from build123d import *

# Parameters (mm, degrees)
SKETCH_1_W               = 40
SKETCH_1_H               = 40.8
SKETCH_1_R               = 8
SKETCH_1_R_2             = 2.025
EXTRUDE_1_DEPTH          = 6
CUT_EXTRUDE_1_DEPTH      = 32.511267826
CUT_EXTRUDE_1_DEPTH_BACK = 32.511267826
SKETCH_2_R               = 1.5


with BuildPart() as part:
    # 草图1 → 凸台-拉伸1 (new body)
    with BuildSketch(Plane(origin=(0, 0, 0), x_dir=(0, 0, -1), z_dir=(1, 0, 0))):
        with Locations((0, 3.2)):
            Rectangle(SKETCH_1_W, SKETCH_1_H)
        Circle(SKETCH_1_R, mode=Mode.SUBTRACT)
        with Locations((-8.838834765, 8.838834765)):
            Circle(SKETCH_1_R_2, mode=Mode.SUBTRACT)
        with Locations((8.838834765, 8.838834765)):
            Circle(SKETCH_1_R_2, mode=Mode.SUBTRACT)
        with Locations((8.838834765, -8.838834765)):
            Circle(SKETCH_1_R_2, mode=Mode.SUBTRACT)
        with Locations((-8.838834765, -8.838834765)):
            Circle(SKETCH_1_R_2, mode=Mode.SUBTRACT)
    extrude(amount=EXTRUDE_1_DEPTH)

    # 草图2 → 切除-拉伸1 (cut, two sides: drawn at the far end of the back side and taken through both)
    with BuildSketch(Plane(origin=(0, 0, 0), x_dir=(1, 0, 0), z_dir=(0, 1, 0)).offset(-CUT_EXTRUDE_1_DEPTH_BACK)):
        with Locations(Location((3, 15, 0), (0, 0, 270))):
            Circle(SKETCH_2_R)
        with Locations(Location((3, -15, 0), (0, 0, 270))):
            Circle(SKETCH_2_R)
    extrude(amount=CUT_EXTRUDE_1_DEPTH + CUT_EXTRUDE_1_DEPTH_BACK, mode=Mode.SUBTRACT)


solid = part.part
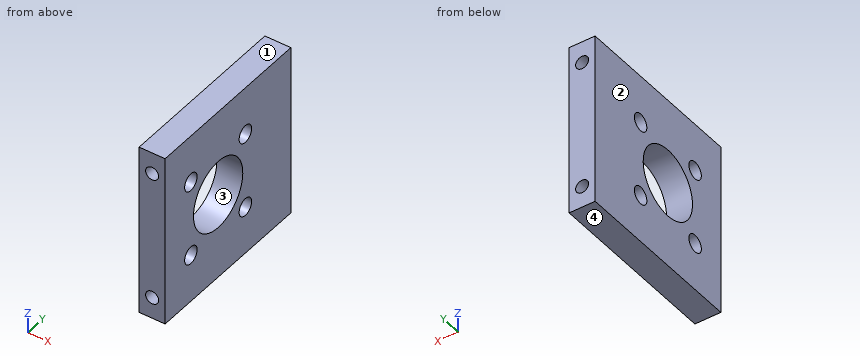
The model under review builds one solid part; all positions refer to its coordinate system, in mm. Face numbers are marked on the shaded views. Give positions to 0.01 mm unless a question says otherwise; leave off trailing zeros. Loops run counter-clockwise (first coordinate to the right, second up) from the corner with the lowest first, then second, coordinate; pieces in that order, holes last. Notation, with made-up numbers: (11.25, 28) -> (36.25, 28) arc R21 cw to (36.25, 40) -> close; hole circle Ø2 at (86, 22.25). An arc over 180 degrees is marked (long way). Answer as a JSON object with one key per item and string values. Group by question number.
Q1. Insertion check: pin 1 (2.5 mm diameter, centred on x = 3, z = 15, fed in from -Y). The pin has a flat end and moves straight along its axis. Give the tip position at first contact, or say it passes through.
Q2. Take a section at C-C (x = 3). Write out the cut boundary in (y, z) (3 decimals), plus the area to 3 significant figures.
Q3. Wall thickness on line 1 along Z through (x, y) = (3.1, 19); line 2 along Y through (x, z) = (2.5, 9); line 3 along Z through (x, y) = (5.45, -9): over which ranges is each line inside the solid? List them lowest first.
Q4. Draft analysis for pull direction Z (two halves, no side actions). For the marked faces 1, 2, 3 and 4, state which applies: pulls with the +Z half, pulls with the -Z half, needs draft (parallel to the pull), parting line crosses it, or undercut.
Q5. Take a section at D-D (x = 5.1). Write out the cut boundary in (y, z) (3 decimals), plus the area to 3 significant figures.
Q6. Take a section at A-A (y = 2.5). Write out the cut boundary in (x, z).
Q7. Take a section at B-B (z = 15). Write out the cut boundary in (x, y).
Answer below:
{
 "1": {"pin 1": "passes through"},
 "2": {"outline": "(-17.2, -20) -> (23.6, -20) -> (23.6, -16.5) -> (-17.2, -16.5) -> close; (-17.2, -13.5) -> (23.6, -13.5) -> (23.6, 13.5) -> (-17.2, 13.5) -> close; (-17.2, 16.5) -> (23.6, 16.5) -> (23.6, 20) -> (-17.2, 20) -> close; hole circle Ø4.05 at (-8.839, -8.839); hole circle Ø4.05 at (-8.839, 8.839); hole circle Ø16 at (0, 0); hole circle Ø4.05 at (8.839, -8.839); hole circle Ø4.05 at (8.839, 8.839)", "area": "1,130 mm2"},
 "3": {"line 1": "z = -20 to -16.5, -13.5 to 13.5, 16.5 to 20", "line 2": "y = -17.2 to -10.86, -6.82 to 6.82, 10.86 to 23.6", "line 3": "z = -20 to -10.86, -6.82 to 6.82, 10.86 to 20"},
 "4": {"face 1": "pulls with the +Z half", "face 2": "needs draft", "face 3": "undercut", "face 4": "pulls with the -Z half"},
 "5": {"outline": "(-17.2, -20) -> (23.6, -20) -> (23.6, 20) -> (-17.2, 20) -> close; hole circle Ø4.05 at (-8.839, -8.839); hole circle Ø4.05 at (-8.839, 8.839); hole circle Ø16 at (0, 0); hole circle Ø4.05 at (8.839, -8.839); hole circle Ø4.05 at (8.839, 8.839)", "area": "1,380 mm2"},
 "6": {"outline": "(0, -20) -> (6, -20) -> (6, -7.6) -> (0, -7.6) -> close; (0, 7.6) -> (6, 7.6) -> (6, 20) -> (0, 20) -> close; hole circle Ø3 at (3, -15); hole circle Ø3 at (3, 15)"},
 "7": {"outline": "(0, -17.2) -> (1.5, -17.2) -> (1.5, 23.6) -> (0, 23.6) -> close; (4.5, -17.2) -> (6, -17.2) -> (6, 23.6) -> (4.5, 23.6) -> close"}
}
